```python
from build123d import *
from build123d.topology import SkipClean

# Parameters (mm, degrees)
SKETCH1_W           = 13.2
SKETCH1_H           = 12.7
BOSS_EXTRUDE1_DEPTH = 9.5
SKETCH2_R           = 3
BOSS_EXTRUDE2_DEPTH = 8.8
SKETCH4_R           = 2.5
CUT_EXTRUDE1_DEPTH  = 2
SKETCH5_R           = 1.5
BOSS_EXTRUDE3_DEPTH = 5
REVOLVE2_ANGLE      = 180
FILLET1_R           = 1
SKETCH6_W           = 0.8
SKETCH6_H           = 2
BOSS_EXTRUDE4_DEPTH = 4
SKETCH7_W           = 1
SKETCH7_H           = 2
CUT_EXTRUDE2_DEPTH  = 26.117773
FILLET2_R           = 0.5
BOSS_EXTRUDE5_START = 5.3
SKETCH8_R           = 2.5
BOSS_EXTRUDE5_DEPTH = 4
BOSS_EXTRUDE6_START = 4
BOSS_EXTRUDE6_DEPTH = 4
FILLET3_R           = 1


# Some blends are built 0.0001 mm under size
with BuildPart() as part:
    # Sketch1 → Boss-Extrude1 (new body)
    with BuildSketch(Plane(origin=(0, 0, 0), x_dir=(1, 0, 0), z_dir=(0, 1, 0))):
        Rectangle(SKETCH1_W, SKETCH1_H)
    extrude(amount=BOSS_EXTRUDE1_DEPTH)

    # Sketch2 → Boss-Extrude2 (add)
    with BuildSketch(Plane(origin=(0, 9.5, 0), x_dir=(1, 0, 0), z_dir=(0, 1, 0))):
        with Locations(Location((0, 0, 0), (0, 0, 270))):
            Circle(SKETCH2_R)
    extrude(amount=BOSS_EXTRUDE2_DEPTH)

    # Sketch4 → Cut-Extrude1 (cut)
    with BuildSketch(Plane(origin=(0, 18.3, 0), x_dir=(1, 0, 0), z_dir=(0, 1, 0))):
        with Locations(Location((0, 0, 0), (0, 0, 270))):
            Circle(SKETCH4_R)
    extrude(amount=-CUT_EXTRUDE1_DEPTH, mode=Mode.SUBTRACT)

    # Sketch5 → Boss-Extrude3 (add)
    with BuildSketch(Plane(origin=(0, 16.3, 0), x_dir=(1, 0, 0), z_dir=(0, 1, 0))):
        with Locations(Location((0, 0, 0), (0, 0, 270))):
            Circle(SKETCH5_R)
    extrude(amount=BOSS_EXTRUDE3_DEPTH)

    # Sketch3 → Revolve2 (revolve)
    with BuildSketch(Plane(origin=(0, 16.3, 0), x_dir=(1, 0, 0), z_dir=(0, 1, 0))):
        with BuildLine():
            Line((0, -2.5), (0, 2.5))
            ThreePointArc((0, 2.5), (-2.5, 0), (0, -2.5))
        make_face()
    revolve(axis=Axis((0, 16.3, 3), (0, 0, -1)), revolution_arc=REVOLVE2_ANGLE)

    # Fillet1
    fillet1_edges = [part.edges().sort_by_distance(p)[0] for p in [
        (0, 21.3, -1.5),
    ]]
    fillet(fillet1_edges, radius=FILLET1_R)

    # Sketch6 → Boss-Extrude4 (add)
    with BuildSketch(Plane.XZ):
        with Locations((-4.7, 2.4)):
            Rectangle(SKETCH6_W, SKETCH6_H)
        with Locations((-4.7, -2.4)):
            Rectangle(SKETCH6_W, SKETCH6_H)
        with Locations((0, -2.4)):
            Rectangle(SKETCH6_W, SKETCH6_H)
        with Locations((0, 2.4)):
            Rectangle(SKETCH6_W, SKETCH6_H)
        with Locations((4.7, 2.4)):
            Rectangle(SKETCH6_W, SKETCH6_H)
        with Locations((4.7, -2.4)):
            Rectangle(SKETCH6_W, SKETCH6_H)
    extrude(amount=BOSS_EXTRUDE4_DEPTH)

    # Sketch7 → Cut-Extrude2 (cut, through all)
    with BuildSketch(Plane.ZY.offset(5.1)):
        with Locations((-2.4, -2.5)):
            Rectangle(SKETCH7_W, SKETCH7_H)
        with Locations((2.4, -2.5)):
            Rectangle(SKETCH7_W, SKETCH7_H)
    extrude(amount=-CUT_EXTRUDE2_DEPTH, mode=Mode.SUBTRACT)

    # Fillet2
    fillet2_edges = [part.edges().sort_by_distance(p)[0] for p in [
        (4.7, -3.5, 2.9),
        (4.7, -3.5, 1.9),
        (4.7, -3.5, -1.9),
        (4.7, -3.5, -2.9),
        (4.7, -1.5, -1.9),
        (4.7, -1.5, 2.9),
        (4.7, -1.5, 1.9),
        (4.7, -1.5, -2.9),
        (0, -1.5, 1.9),
        (0, -1.5, 2.9),
        (0, -3.5, 2.9),
        (0, -3.5, 1.9),
        (0, -3.5, -1.9),
        (0, -3.5, -2.9),
        (0, -1.5, -2.9),
        (0, -1.5, -1.9),
        (-4.7, -3.5, 2.9),
        (-4.7, -1.5, 2.9),
        (-4.7, -3.5, 1.9),
        (-4.7, -1.5, 1.9),
        (-4.7, -1.5, -1.9),
        (-4.7, -1.5, -2.9),
        (-4.7, -3.5, -1.9),
        (-4.7, -3.5, -2.9),
        (0, -4, -1.4),
        (0, -4, -3.4),
        (4.7, -4, -1.4),
        (4.7, -4, -3.4),
        (4.7, -4, 1.4),
        (4.7, -4, 3.4),
        (0, -4, 3.4),
        (0, -4, 1.4),
        (-4.7, -4, 3.4),
        (-4.7, -4, 1.4),
        (-4.7, -4, -1.4),
        (-4.7, -4, -3.4),
    ]]
    fillet(fillet2_edges, radius=FILLET2_R - 0.0001)  # a hair under: the kernel refuses the full size

    # Sketch8 → Boss-Extrude5 (add)
    with BuildSketch(Plane(origin=(0, 18.3, 0), x_dir=(1, 0, 0), z_dir=(0, 1, 0)).offset(BOSS_EXTRUDE5_START)):
        with Locations(Location((0, 0, 0), (0, 0, 270))):
            Circle(SKETCH8_R)
    extrude(amount=-BOSS_EXTRUDE5_DEPTH)

    # Sketch9 → Boss-Extrude6 (add)
    with SkipClean():  # the faces are left unmerged after this step: merging them gives an invalid solid
        with BuildSketch(Plane(origin=(0, 23.6, 0), x_dir=(1, 0, 0), z_dir=(0, 1, 0)).offset(BOSS_EXTRUDE6_START)):
            with BuildLine():
                Line((-1, -2.291288), (-1, 2.291288))
                ThreePointArc((-1, 2.291288), (0, 2.5), (1, 2.291288))
                Line((1, 2.291288), (1, -2.291288))
                ThreePointArc((1, -2.291288), (0, -2.5), (-1, -2.291288))
            make_face()
        extrude(amount=-BOSS_EXTRUDE6_DEPTH)

    # Fillet3
    # the kernel refuses this fillet: 1 mm, written as the material it adds along each edge
    with BuildSketch(Plane(origin=(1, 23.6, -4.791288), x_dir=(1, 0, 0), z_dir=(0, 0, 1))) as fillet3_piece_1_section:
        with BuildLine():
            CenterArc((FILLET3_R, FILLET3_R), FILLET3_R, 180, 90)
            Line((0, FILLET3_R), (0, 0))
            Line((0, 0), (FILLET3_R, 0))
        make_face()
    fillet3_piece_1 = extrude(amount=9.582576, mode=Mode.PRIVATE)
    fillet3_piece_1 = fillet3_piece_1 & Plane(origin=(0, 23.834238, 0), x_dir=(0, 0, 1), z_dir=(0, 1, 0)) * Cylinder(2.5, 24, mode=Mode.PRIVATE)
    add(fillet3_piece_1)
    with BuildSketch(Plane(origin=(-1, 23.6, 4.791288), x_dir=(-1, 0, 0), z_dir=(0, 0, -1))) as fillet3_piece_2_section:
        with BuildLine():
            CenterArc((FILLET3_R, FILLET3_R), FILLET3_R, 180, 90)
            Line((0, FILLET3_R), (0, 0))
            Line((0, 0), (FILLET3_R, 0))
        make_face()
    fillet3_piece_2 = extrude(amount=9.582576, mode=Mode.PRIVATE)
    fillet3_piece_2 = fillet3_piece_2 & Plane(origin=(0, 23.834238, 0), x_dir=(0, 0, 1), z_dir=(0, 1, 0)) * Cylinder(2.5, 24, mode=Mode.PRIVATE)
    add(fillet3_piece_2)


solid = part.part
```
For this review, take the finished solid that the model builds, in its own axes (mm). A direction names the side the tool comes from. Round coordinates to 2 decimals unless told otherwise and drop trailing zeros. Order: outer loops, then holes, each group sorted by start corner. A loop starts at its lowest first (then second) coordinate and runs counter-clockwise, first axis right, second up.
Q1. We need section B-B, the plane x = 0. State how many separate pieces and enclosed holes the cut face has, plus the area to 3 significant figures.
Findings below:
separate pieces: 1
enclosed holes: 2
area: 228 mm2
Q2. We need section A-A, the plane z = 0. Give the boundary of the cut face in (x, y).
Findings below:
outline: (-6.6, 0) - (6.6, 0) - (6.6, 9.5) - (3, 9.5) - (3, 18.3) - (2.5, 18.3) - (2.5, 16.3) arc R2.5 ccw to (1.5, 18.3) - (1.5, 19.6) - (2.5, 19.6) - (2.5, 23.6) - (2, 23.6) arc R1 cw to (1, 24.6) - (1, 27.6) - (-1, 27.6) - (-1, 24.6) arc R1 cw to (-2, 23.6) - (-2.5, 23.6) - (-2.5, 19.6) - (-1.5, 19.6) - (-1.5, 18.3) arc R2.5 ccw to (-2.5, 16.3) - (-2.5, 18.3) - (-3, 18.3) - (-3, 9.5) - (-6.6, 9.5) - close
Q3. We need section D-D, the plane y = 13.5. Give the boundary of the cut face in (x, z), plus the area to 3 significant figures.
Findings below:
outline: circle Ø6 at (0, 0)
area: 28.3 mm2
Q4. Wall thickness on line 1 (X direction, y = 17.8, z = 0); line 2 (X direction, y = -0.5, z = -2.5); line 3 (Y direction, x = 0.75, z = 0): over which ranges is each line inside the solid? List them lowest first.
Findings below:
line 1: x = -3 to -2.5, -2 to 2, 2.5 to 3
line 2: x = -5.1 to -4.3, -0.4 to 0.4, 4.3 to 5.1
line 3: y = 0 to 27.6
Q5. We need section C-C, the plane y = 25. Give the boundary of the cut face in (x, z).
Findings below:
outline: (-1, -2.29) arc R2.5 ccw to (1, -2.29) - (1, 2.29) arc R2.5 ccw to (-1, 2.29) - close
Q6. Machinability: for faces 4 (the flat face through (-0.4, -1.5, 1.9)), 5 (the flat face through (-4.7, -1.7, 1.4)), 6 (the flat face through (-4.7, -2.5, 2.9)), 7 (the flat face through (4.7, -1.7, 3.4)), which of the approach directions +Z, -Z, +X, -X, +Y, -Y give a long, thin tool a straight path to every point of the face, cutting with its end or side? Answer none if there is none.
Findings below:
face 4: +Z, -Z, -Y
face 5: +X, -X, -Y
face 6: +X, -X
face 7: +Z, +X, -X, -Y
Q7. Mouldability with a two-part tool opening along Y and no side actions: class faces 1 (the flat face through (-4.7, -1.7, -3.4)), 2 (the cylindrical face through (0.45, 18.94, 1.43)), 3 (the flat face through (2, 18.3, -2)) as pulls with the +Y half, pulls with the -Y half, needs draft (parallel to the pull), parting line crosses it, or undercut.
Findings below:
face 1: needs draft
face 2: undercut
face 3: pulls with the +Y half
Q8. Insertion check: P1, Ø1, axis at y = -2.5, z = -2.5, coming from the +X side; P2, Ø1, axis at y = 23, z = 1, coming from the -X side; P3, Ø3, axis at x = 2, y = 12, coming from the +Z side. Each pin has a flat end and moves straight along its axis. Give the tip position at first contact, or say it passes through.
Findings below:
P1: stops at x = 5.1
P2: stops at x = -2.45
P3: stops at z = 2.96
